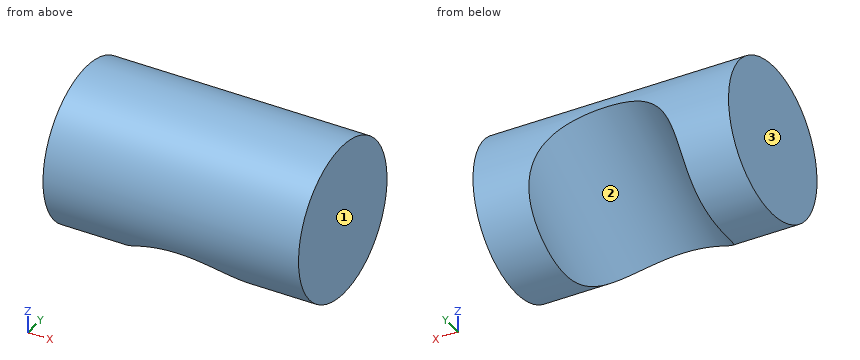
```python
from build123d import *

# Parameters (mm, degrees)
F0_R          = 14.995
F1_DEPTH      = 25
F1_DEPTH_BACK = 25
F2_R          = 15
F3_DEPTH      = 25
F3_DEPTH_BACK = 25
F5_ANGLE      = 30


with BuildPart() as f1:
    # F0 (on Right) → F1 (new body, two sides)
    with BuildSketch(Plane.YZ) as f1_sk:
        Circle(F0_R)
    extrude(amount=F1_DEPTH)
    extrude(f1_sk.sketch, amount=-F1_DEPTH_BACK)

    # F2 (on Front) → F3 (cut, two sides)
    with BuildSketch(Plane.XZ) as f3_sk:
        with Locations((0, -15)):
            Circle(F2_R)
    extrude(amount=-F3_DEPTH, mode=Mode.SUBTRACT)
    extrude(f3_sk.sketch, amount=F3_DEPTH_BACK, mode=Mode.SUBTRACT)


with BuildPart() as f1_1:
    # F5: moved
    add(f1.part.rotate(Axis((31.3068032265, 0, 0), (1, 0, 0)), F5_ANGLE))


solid = f1_1.part
```
Here's how the part is built. I have some questions about the finished solid (model axes, mm). Face numbers are marked on the shaded views. Round coordinates to 2 decimals unless told otherwise and drop trailing zeros. Loops run counter-clockwise (first coordinate to the right, second up) from the corner with the lowest first, then second, coordinate; pieces in that order, holes last. Notation, with made-up numbers: (-28.5, 59.5) -> (3.5, 59.5) arc R5 ccw to (3.5, 68.5) -> close; hole circle Ø4 at (7, -33). An arc over 180 degrees is marked (long way). Answer as CSV lines item,"result".
1. Thinking about a two-plate mould opening in X: for the marked faces 1, 2 and 3, which applies, released by +X, released by -X, zero draft, split by the parting line, or undercut?
Final values:
face 1,"released by +X"
face 2,"undercut"
face 3,"released by -X"
2. If we section it at A-A on z = 12.75: Please give me the cut outline in (x, y), plus the area to 3 significant figures.
Final values:
outline,"(-25, -7.89) -> (25, -7.89) -> (25, 7.89) -> (-25, 7.89) -> close"
area,"789 mm^2"
3. For pin 1 (1.5 mm diameter, centred on x = 2, y = -6.5, fed in from +Z); pin 2 (1.5 mm diameter, centred on x = 12, z = 8, fed in from -Y); pin 3 (5 mm diameter, centred on x = -14, y = -4.5, fed in from -Z), each with a flat end and sliding along its axis, tell me the tip position at first contact or that it passes through.
Final values:
pin 1,"stops at z = 13.85"
pin 2,"stops at y = -13.13"
pin 3,"stops at z = -14.85"
4. If I drill on L1, parallel to X at y = 10.75, z = 4.25; L2, parallel to X at y = 10, z = -10.75; L3, parallel to Y at x = 15.5, z = 0.25, over which ranges is the centre line in solid material (lowest first)?
Final values:
L1,"x = -25 to -6.93, 6.93 to 25"
L2,"x = -25 to -14.98, 14.98 to 25"
L3,"y = -14.99 to 14.99"
